Source: CAD feature listing. Evaluate the final solid. Frame: model axes, mm. A direction names the side the tool comes from. Give positions to 0.01 mm unless a question says otherwise; leave off trailing zeros. Loops run counter-clockwise (first coordinate to the right, second up) from the corner with the lowest first, then second, coordinate; pieces in that order, holes last. Notation, with made-up numbers: M 68.25,-16 L 72.25,-16 A11 cw 72.25,-8 Z; hole C 56.25,46.5 d3. An arc over 180 degrees is marked long. Put each result on its own line as item: value.
from build123d import *

# Parameters (mm, degrees)
F0_R     = 2
F1_DEPTH = 4


# Not quite as in the source:
# - a feature names something its author has since deleted; it is built from what else it names


with BuildPart() as f1:
    # F0 (on Top) → F1 (new body)
    with BuildSketch(Plane.XY):
        Polygon((-235, 194), (-235, 190), (-235, -170), (-235, -190), (-235, -194), (235, -194), (235, -190), (235, -28), (230, -28), (230, 0), (230, 28), (235, 28), (235, 190), (235, 194), align=None)
        with Locations((-200, -180)):
            Circle(F0_R, mode=Mode.SUBTRACT)
        with Locations((-225, -150)):
            Circle(F0_R, mode=Mode.SUBTRACT)
        with Locations((-225, 0)):
            Circle(F0_R, mode=Mode.SUBTRACT)
        with BuildLine():
            Line((110, -161.9999999998), (-177, -162))
            ThreePointArc((-177, -162), (-198.2132034356, -153.2132034356), (-207, -132))
            Line((-207, -132), (-207, 0))
            Line((-207, 0), (-207, 132))
            ThreePointArc((-207, 132), (-198.2132034356, 153.2132034356), (-177, 162))
            Line((-177, 162), (110, 161.9999999998))
            ThreePointArc((110, 161.9999999998), (131.2132034356, 153.2132034354), (140, 131.9999999998))
            Line((140, 131.9999999998), (140, 0))
            Line((140, 0), (140, -131.9999999998))
            ThreePointArc((140, -131.9999999998), (131.2132034356, -153.2132034354), (110, -161.9999999998))
        make_face(mode=Mode.SUBTRACT)
        with Locations((0, -180)):
            Circle(F0_R, mode=Mode.SUBTRACT)
        with Locations((175, -150)):
            Circle(F0_R, mode=Mode.SUBTRACT)
        with Locations((205, -180)):
            Circle(F0_R, mode=Mode.SUBTRACT)
        with Locations((175, 0)):
            Circle(F0_R, mode=Mode.SUBTRACT)
        with Locations((-225, 150)):
            Circle(F0_R, mode=Mode.SUBTRACT)
        with Locations((-200, 180)):
            Circle(F0_R, mode=Mode.SUBTRACT)
        with Locations((0, 180)):
            Circle(F0_R, mode=Mode.SUBTRACT)
        with Locations((175, 150)):
            Circle(F0_R, mode=Mode.SUBTRACT)
        with Locations((205, 180)):
            Circle(F0_R, mode=Mode.SUBTRACT)
    extrude(amount=F1_DEPTH)


solid = f1.part
1. Draft query along X for faces 1 (the flat face through (153, 3, 4)), 2 (the cylindrical face through (-197.979, -153.445, 1.972)). Return one class per face: pulls with the +X half, pulls with the -X half, needs draft (parallel to the pull), parting line crosses it, or undercut.
Found:
face 1: needs draft
face 2: undercut
2. Section query A-A (x = 59.5). Output: boundary loops of the cut face in (y, z), plus the area to 3 significant figures.
Found:
outline: M -194,0 L -162,0 L -162,4 L -194,4 Z; M 162,0 L 194,0 L 194,4 L 162,4 Z
area: 256 mm^2
3. Section query B-B (y = -22.5). Output: boundary loops of the cut face in (x, z).
Found:
outline: M -235,0 L -207,0 L -207,4 L -235,4 Z; M 140,0 L 230,0 L 230,4 L 140,4 Z
4. Access query for faces 3 (the flat face through (153, 3, 0)), 4 (the cylindrical face through (131.445, -152.979, 1.972)). Directions: +Z, -Z, +X, -X, +Y, -Y. A direction counts if a zero-diameter tool reaches every point of the face in a straight line with its end or side. Return the directions, or none.
Found:
face 3: -Z, +X, -X, +Y, -Y
face 4: +Z, -Z
5. Contact query for flat-ended pins moving along their axis: P1, Ø3.5, axis at x = 175, y = 150, coming from the +Z side; P2, Ø1.2, axis at y = 0, z = 1.5, coming from the +X side. Output: stop coordinate, or through.
Found:
P1: through
P2: x = 230
6. Material intervals for line 1 (Y direction, x = -225, z = 2.2); line 2 (X direction, y = -180, z = 3.1); line 3 (Y direction, x = -7, z = 2.05), sorted ascending. Write a range as from..to.
Found:
line 1: -194..-152, -148..-2, 2..148, 152..194
line 2: -235..-202, -198..-2, 2..203, 207..235
line 3: -194..-162, 162..194
7. Section query C-C (z = 2.1). State how many separate pieces and enclosed holes the cut face has, plus the area to 3 significant figures.
Found:
separate pieces: 1
enclosed holes: 13
area: 70,300 mm^2
